from build123d import *

# Parameters (mm, degrees)
SKETCH1_R           = 3.25
SKETCH1_R_2         = 3.85
SKETCH1_R_3         = 2
BOSS_EXTRUDE1_DEPTH = 5


with BuildPart() as part:
    # Sketch1 → Boss-Extrude1 (new body)
    with BuildSketch(Plane.XY):
        with BuildLine():
            ThreePointArc((0, -30.4), (30.4, 0), (0, 30.4))
            ThreePointArc((0, 30.4), (-30.4, 0), (0, -30.4))
        make_face()
        with Locations((0, 25)):
            Circle(SKETCH1_R, mode=Mode.SUBTRACT)
        with Locations((17.67766953, 17.67766953)):
            Circle(SKETCH1_R_2, mode=Mode.SUBTRACT)
        with Locations((17.67766953, -17.67766953)):
            Circle(SKETCH1_R_2, mode=Mode.SUBTRACT)
        with Locations((-17.67766953, -17.67766953)):
            Circle(SKETCH1_R_2, mode=Mode.SUBTRACT)
        with Locations((-17.67766953, 17.67766953)):
            Circle(SKETCH1_R_2, mode=Mode.SUBTRACT)
        with Locations((24, 0)):
            Circle(SKETCH1_R_3, mode=Mode.SUBTRACT)
        with Locations((-24, 0)):
            Circle(SKETCH1_R_3, mode=Mode.SUBTRACT)
    extrude(amount=BOSS_EXTRUDE1_DEPTH)


solid = part.part
Verification items for the finished model (mm, model axes). Round coordinates to 2 decimals unless told otherwise and drop trailing zeros. Loops run counter-clockwise (first coordinate to the right, second up) from the corner with the lowest first, then second, coordinate; pieces in that order, holes last. Notation, with made-up numbers: (-1, -2.5) - (5, -2.5) arc R21 ccw to (5, 23.5) - close; hole circle Ø6 at (85, 2.5). An arc over 180 degrees is marked (long way). Use one line per item in the form item = value.
1. Section check B-B on y = 0. Record the cut outline in (x, z).
A:
outline = (-30.4, 0) - (-26, 0) - (-26, 5) - (-30.4, 5) - close; (-22, 0) - (22, 0) - (22, 5) - (-22, 5) - close; (26, 0) - (30.4, 0) - (30.4, 5) - (26, 5) - close
2. Gauge pin test, flat ends, axial feed: pin 1 Ø4.5 at (x, y) = (-17.68, -17.68) entering from -Z; pin 2 Ø1.5 at (x, z) = (5.5, 4) entering from +Y. Record the tip position at first contact, or that the pin passes through.
A:
pin_1 = through
pin_2 = 30.03
3. Section check D-D on z = 1. Record the cut outline in (x, y).
A:
outline = circle Ø60.8 at (0, 0); hole circle Ø4 at (-24, 0); hole circle Ø7.7 at (-17.68, -17.68); hole circle Ø7.7 at (-17.68, 17.68); hole circle Ø6.5 at (0, 25); hole circle Ø7.7 at (17.68, -17.68); hole circle Ø7.7 at (17.68, 17.68); hole circle Ø4 at (24, 0)
4. Scan lines: probe 1 along Y at (x, z) = (-21, 3.15); probe 2 along X at (y, z) = (14.5, 4.75); probe 3 along Y at (x, z) = (-20.5, 1.8). Record each from-to range of solid material in increasing order.
A:
probe_1 = -21.98 to -19.62, -15.73 to 15.73, 19.62 to 21.98
probe_2 = -26.72 to -19.85, -15.5 to 15.5, 19.85 to 26.72
probe_3 = -22.45 to -20.3, -15.06 to 15.06, 20.3 to 22.45
5. Section check C-C on y = 25. Record the cut outline in (x, z).
A:
outline = (-17.3, 0) - (-3.25, 0) - (-3.25, 5) - (-17.3, 5) - close; (3.25, 0) - (17.3, 0) - (17.3, 5) - (3.25, 5) - close
6. Section check A-A on x = 0. Record the cut outline in (y, z).
A:
outline = (-30.4, 0) - (21.75, 0) - (21.75, 5) - (-30.4, 5) - close; (28.25, 0) - (30.4, 0) - (30.4, 5) - (28.25, 5) - close
7. Draft check along X on faces 1 (the cylindrical face through (-25.633, 16.343, 2.465)), 2 (the flat face through (0, 0, 0)), 3 (the cylindrical face through (16.84, 13.92, 2.46)). Enter one of: pulls with the +X half, pulls with the -X half, needs draft (parallel to the pull), parting line crosses it, or undercut.
A:
face_1 = parting line crosses it
face_2 = needs draft
face_3 = undercut
